from build123d import *

# Parameters (mm, degrees)
SKETCH1_W                  = 450
SKETCH1_H                  = 167.8324167
BOSS_EXTRUDE1_DEPTH        = 1.6002
F_10_CLEARANCE_HOLE1_D     = 5.1054
F_10_CLEARANCE_HOLE1_DEPTH = 129.53
F_10_CLEARANCE_HOLE1_TIP   = 1.533816902
SKETCH4_R                  = 7.5
CUT_EXTRUDE1_DEPTH         = 2.6002
SKETCH5_W                  = 355.6
SKETCH5_H                  = 101.6
CUT_EXTRUDE2_DEPTH         = 2.6002
FILLET1_R                  = 10
F_10_CLEARANCE_HOLE2_D     = 5.1054
MIRROR2_COPY_1_D           = 5.1054


with BuildPart() as part:
    # Sketch1 → Boss-Extrude1 (new body)
    with BuildSketch(Plane(origin=(0, 0, 0), x_dir=(0, 0, -1), z_dir=(1, 0, 0))):
        with Locations((0, -3.9624)):
            Rectangle(SKETCH1_W, SKETCH1_H)
    extrude(amount=BOSS_EXTRUDE1_DEPTH)

    # #10 Clearance Hole1
    with Locations(Plane(origin=(1.6002, 0, 0), x_dir=(0, 0, -1), z_dir=(1, 0, 0))):
        with Locations((-190, 73.59110835), (35, 73.59110835), (-35, -73.59110835), (-190, -73.59110835), (190, 73.59110835), (190, -73.59110835)):
            Hole(F_10_CLEARANCE_HOLE1_D / 2, depth=F_10_CLEARANCE_HOLE1_DEPTH)
            with Locations((0, 0, -(F_10_CLEARANCE_HOLE1_DEPTH + F_10_CLEARANCE_HOLE1_TIP / 2))):  # 118° drill point
                Cone(0, F_10_CLEARANCE_HOLE1_D / 2, F_10_CLEARANCE_HOLE1_TIP, mode=Mode.SUBTRACT)

    # Sketch4 → Cut-Extrude1 (cut, through all)
    with BuildSketch(Plane(origin=(1.6002, 0, 0), x_dir=(0, 0, -1), z_dir=(1, 0, 0))):
        with Locations((-206.5, -56.5321)):
            Circle(SKETCH4_R)
    extrude(amount=-CUT_EXTRUDE1_DEPTH, mode=Mode.SUBTRACT)

    # Sketch5 → Cut-Extrude2 (cut, through all)
    with BuildSketch(Plane(origin=(1.6002, 0, 0), x_dir=(0, 0, -1), z_dir=(1, 0, 0))):
        Rectangle(SKETCH5_W, SKETCH5_H)
    extrude(amount=-CUT_EXTRUDE2_DEPTH, mode=Mode.SUBTRACT)

    # Fillet1
    fillet1_edges = [part.edges().sort_by_distance(p)[0] for p in [
        (0.8001, -50.8, 177.8),
        (0.8001, 50.8, 177.8),
        (0.8001, 50.8, -177.8),
        (0.8001, -50.8, -177.8),
    ]]
    fillet(fillet1_edges, radius=FILLET1_R)

    # #10 Clearance Hole2 (through all)
    with Locations(Plane(origin=(1.6002, 0, 0), x_dir=(0, 0, -1), z_dir=(1, 0, 0))):
        with Locations((197.627, 40)):
            f_10_clearance_hole2 = Hole(F_10_CLEARANCE_HOLE2_D / 2)

    # Mirror1: #10 Clearance Hole2 across plane
    add(f_10_clearance_hole2.mirror(Plane.ZX), mode=Mode.SUBTRACT)

    # Mirror2: #10 Clearance Hole2 across plane
    add(f_10_clearance_hole2.mirror(Plane.XY), mode=Mode.SUBTRACT)

    # Mirror2 copy 1 (through all)
    with Locations(Plane(origin=(1.6002, 0, 0), x_dir=(0, 0, 1), z_dir=(1, 0, 0))):
        with Locations((197.627, 40)):
            Hole(MIRROR2_COPY_1_D / 2)


solid = part.part
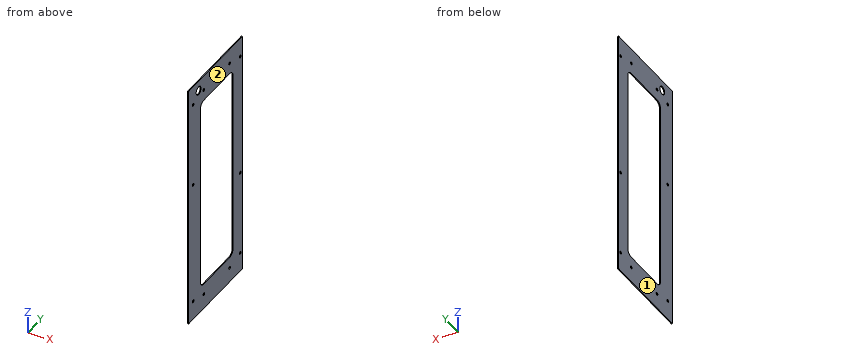
Input: part model. Units: mm. Frame: model coordinates. Face numbers are marked on the shaded views. Round coordinates to 2 decimals unless told otherwise and drop trailing zeros. Order: outer loops, then holes, each group sorted by start corner. A loop starts at its lowest first (then second) coordinate and runs counter-clockwise, first axis right, second up. Notation, with made-up numbers: (46.5, 54.25) - (94.5, 54.25) arc R5 cw to (94.5, 60.25) - close; hole circle Ø1 at (-21, 41.25). An arc over 180 degrees is marked (long way). Answer as a JSON object with one key per item and string values. Group by question number.
(1) Cut plane B-B (y = -24). Return loops of the section in (x, z), then the cut area to 3 significant figures.
(2) Cut plane A-A (z = 206.5). Return loops of the section in (x, y).
(3) Cut plane C-C (x = 1). Count the separate pieces of the cut face and the enclosed holes in it, then the cut area to 3 significant figures.
(4) Draft query along X for the marked faces 1 and 2. Return one class per face: released by +X, released by -X, zero draft, split by the parting line, or undercut.
(5) Material intervals for probe 1 along Y at (x, z) = (1.3, -190); probe 2 along Y at (x, z) = (0.2, -49); probe 3 along Y at (x, z) = (0.45, -35), sorted ascending. Write a range as from..to.
Here are the results:
{
 "1": {"outline": "(0, -225) - (1.6, -225) - (1.6, -177.8) - (0, -177.8) - close; (0, 177.8) - (1.6, 177.8) - (1.6, 225) - (0, 225) - close", "area": "151 mm^2"},
 "2": {"outline": "(0, -87.88) - (1.6, -87.88) - (1.6, -64.03) - (0, -64.03) - close; (0, -49.03) - (1.6, -49.03) - (1.6, 79.95) - (0, 79.95) - close"},
 "3": {"separate pieces": "1", "enclosed holes": "12", "area": "39,100 mm^2"},
 "4": {"face 1": "released by -X", "face 2": "released by +X"},
 "5": {"probe 1": "y = -87.88..-76.14, -71.04..71.04, 76.14..79.95", "probe 2": "y = -87.88..-50.8, 50.8..79.95", "probe 3": "y = -87.88..-50.8, 50.8..71.04, 76.14..79.95"}
}
